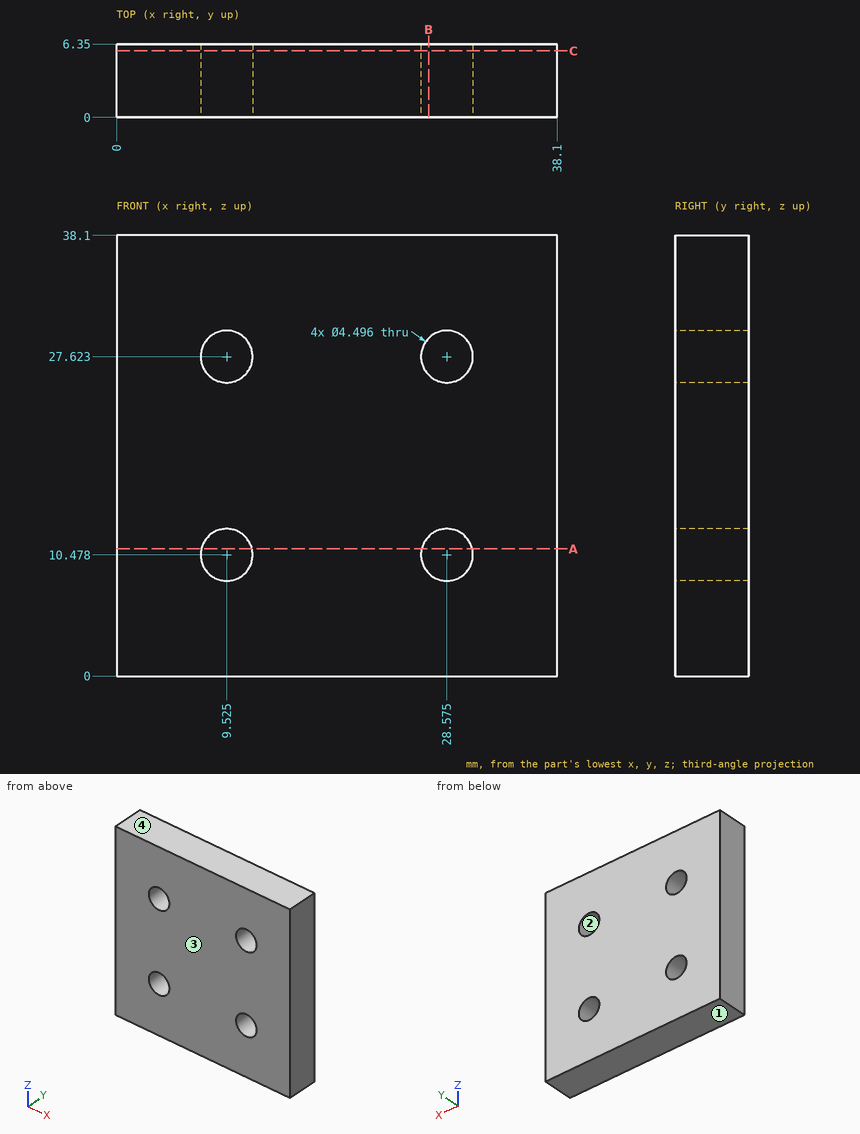
Geometry check sheet. Reference: drawing and pictorial views, mm from the part's lowest x, y, z. Give positions to 0.01 mm unless a question says otherwise; leave off trailing zeros. Order: outer loops, then holes, each group sorted by start corner. A loop starts at its lowest first (then second) coordinate and runs counter-clockwise, first axis right, second up. Notation, with made-up numbers: (11, -13) - (45, -13) arc R13 ccw to (45, -2) - close; hole circle Ø6 at (-26, 15.25). An arc over 180 degrees is marked (long way). Answer as CSV lines item,"result".
1. Scan lines: probe 1 along X at (y, z) = (1.5, 28); probe 2 along Z at (x, y) = (27, 3.5) (1 decimal). Record each from-to range of solid material in increasing order. Write a range as from..to.
Result sheet:
probe 1,"0..7.31, 11.74..26.36, 30.79..38.1"
probe 2,"0..8.9, 12.1..26, 29.2..38.1"
2. Section check C-C (y = 5.75). Record the boundary of the cut face in (x, z) (1 decimal), then the cut area to 3 significant figures.
Result sheet:
outline,"(0, 0) - (38.1, 0) - (38.1, 38.1) - (0, 38.1) - close; hole circle Ø4.5 at (9.5, 10.5); hole circle Ø4.5 at (9.5, 27.6); hole circle Ø4.5 at (28.6, 10.5); hole circle Ø4.5 at (28.6, 27.6)"
area,"1,390 mm²"
3. Section check B-B (x = 27). Record the boundary of the cut face in (y, z).
Result sheet:
outline,"(0, 0) - (6.35, 0) - (6.35, 8.87) - (0, 8.87) - close; (0, 12.08) - (6.35, 12.08) - (6.35, 26.02) - (0, 26.02) - close; (0, 29.23) - (6.35, 29.23) - (6.35, 38.1) - (0, 38.1) - close"
4. Section check A-A (z = 11). Record the boundary of the cut face in (x, y).
Result sheet:
outline,"(0, 0) - (7.34, 0) - (7.34, 6.35) - (0, 6.35) - close; (11.71, 0) - (26.39, 0) - (26.39, 6.35) - (11.71, 6.35) - close; (30.76, 0) - (38.1, 0) - (38.1, 6.35) - (30.76, 6.35) - close"
5. Mould release check, pull along Z, two halves, no side actions. Record for the marked faces 1, 2, 3 and 4: released by +Z, released by -Z, zero draft, split by the parting line, or undercut.
Result sheet:
face 1,"released by -Z"
face 2,"undercut"
face 3,"zero draft"
face 4,"released by +Z"
